from build123d import *

# Parameters (mm, degrees)
AUFSATZ_LINEAR_AUSTRAGEN1_DEPTH = 105
M5_GEWINDEBOHRUNG1_D            = 4.2
M5_GEWINDEBOHRUNG1_DEPTH        = 14
M5_GEWINDEBOHRUNG1_TIP          = 1.2618073
M5_GEWINDEBOHRUNG2_D            = 4.2
M5_GEWINDEBOHRUNG2_DEPTH        = 14
M5_GEWINDEBOHRUNG2_TIP          = 1.2618073
M5_GEWINDEBOHRUNG3_D            = 4.2


with BuildPart() as part:
    # Skizze1 → Aufsatz-Linear austragen1 (new body, symmetric)
    with BuildSketch(Plane.XY):
        Polygon((-40, 0), (40, 0), (40, 10), (10, 10), (10, 4), (-10, 4), (-10, 10), (-40, 10), align=None)
    extrude(amount=AUFSATZ_LINEAR_AUSTRAGEN1_DEPTH, both=True)

    # M5 Gewindebohrung1
    with Locations(Plane.XY.offset(105)):
        with Locations((-30, 4), (30, 4)):
            Hole(M5_GEWINDEBOHRUNG1_D / 2, depth=M5_GEWINDEBOHRUNG1_DEPTH)
            with Locations((0, 0, -(M5_GEWINDEBOHRUNG1_DEPTH + M5_GEWINDEBOHRUNG1_TIP / 2))):  # 118° drill point
                Cone(0, M5_GEWINDEBOHRUNG1_D / 2, M5_GEWINDEBOHRUNG1_TIP, mode=Mode.SUBTRACT)

    # M5 Gewindebohrung2
    with Locations(Plane(origin=(0, 0, -105), x_dir=(-1, 0, 0), z_dir=(0, 0, -1))):
        with Locations((-25, 5), (25, 5)):
            Hole(M5_GEWINDEBOHRUNG2_D / 2, depth=M5_GEWINDEBOHRUNG2_DEPTH)
            with Locations((0, 0, -(M5_GEWINDEBOHRUNG2_DEPTH + M5_GEWINDEBOHRUNG2_TIP / 2))):  # 118° drill point
                Cone(0, M5_GEWINDEBOHRUNG2_D / 2, M5_GEWINDEBOHRUNG2_TIP, mode=Mode.SUBTRACT)

    # M5 Gewindebohrung3 (through all)
    with Locations(Plane(origin=(0, 10, 0), x_dir=(1, 0, 0), z_dir=(0, 1, 0))):
        with Locations((25, -75), (-25, -75), (-25, -45), (-25, -15), (-25, 15), (-25, 45), (-25, 75), (25, 75), (25, 45), (25, 15), (25, -15), (25, -45)):
            Hole(M5_GEWINDEBOHRUNG3_D / 2)


solid = part.part
Verification items for the finished model (mm, model axes). A direction names the side the tool comes from. Coordinates: 2 decimals unless noted, no trailing zeros. Write each loop counter-clockwise with the first axis right and the second up, starting at its lowest first coordinate (ties: lowest second). Pieces come first, ordered by that corner, then holes. Notation, with made-up numbers: M 84,45.5 L 90,45.5 A21 ccw 90,65.5 Z; hole C 6.5,-35.5 d9. An arc over 180 degrees is marked long. One line per question, with ' | ' between items.
1) Depth check by flat-ended pin: pin 1 Ø3.5 at (x, y) = (30, 4) entering from +Z; pin 2 Ø4 at (x, y) = (-25, 5) entering from -Z. Enter the tip coordinate at first touch or a pass-through.
Solutions:
pin 1: z = 90.79 | pin 2: z = -90.94
2) Material ranges on L1, parallel to X at y = 7.5, z = 75; L2, parallel to X at y = 7.25, z = 53; L3, parallel to X at y = 3.25, z = 95.5, recorded low to high.
Solutions:
L1: -40 to -27.1, -22.9 to -10, 10 to 22.9, 27.1 to 40 | L2: -40 to -10, 10 to 40 | L3: -40 to -31.96, -28.04 to 28.04, 31.96 to 40
3) Sectioned sample at A-A on z = 15. Record the cut outline in (x, y), then the cut area to 3 significant figures.
Solutions:
outline: M -40,0 L -27.1,0 L -27.1,10 L -40,10 Z; M -22.9,0 L 22.9,0 L 22.9,10 L 10,10 L 10,4 L -10,4 L -10,10 L -22.9,10 Z; M 27.1,0 L 40,0 L 40,10 L 27.1,10 Z | area: 596 mm^2
4) Sectioned sample at B-B on z = 63. Record the cut outline in (x, y).
Solutions:
outline: M -40,0 L 40,0 L 40,10 L 10,10 L 10,4 L -10,4 L -10,10 L -40,10 Z
5) Access from +Z, -Z, +X, -X, +Y, -Y to the whole of each face (thin tool, end or side, straight path). Record for faces 1 (the face through (-1, 0, 1)), 2 (the face through (24.031, 4.93, 76.863)), 3 (the face through (27.003, 5.631, -97.902)), 4 (the face through (0, 4, 1)), 5 (the face through (-27.9, 4.09, 97.9)).
Solutions:
face 1: +Z, -Z, +X, -X, -Y | face 2: +Y, -Y | face 3: -Z | face 4: +Z, -Z, +Y | face 5: +Z
6) Release check for a two-part mould opening along X. For faces 6 (the face through (-1, 3, -105)), 7 (the face through (-25.2, 5.31, -89.96)), 8 (the face through (40, 5, 1)) record: +X half, -X half, draft (parallel to the pull), parting line (faces both ways), or undercut.
Solutions:
face 6: draft | face 7: undercut | face 8: +X half
